Here's how the part is built. I have some questions about the finished solid (model axes, mm). A direction names the side the tool comes from. Give positions to 0.01 mm unless a question says otherwise; leave off trailing zeros. Loops run counter-clockwise (first coordinate to the right, second up) from the corner with the lowest first, then second, coordinate; pieces in that order, holes last. Notation, with made-up numbers: (61, 27.5) - (72, 27.5) arc R13 ccw to (72, 48.5) - close; hole circle Ø1 at (-30.5, -10). An arc over 180 degrees is marked (long way). Put each result on its own line as item: value. Start each with the question number.
from build123d import *

# Parameters (mm, degrees)
ESQUISSE1_W             = 5
ESQUISSE1_H             = 40
BOSS_EXTRU_1_DEPTH      = 10
ESQUISSE2_R             = 2.6
ENL_V_MAT_EXTRU_1_DEPTH = 10
ESQUISSE3_W             = 5
ESQUISSE3_H             = 40
BOSS_EXTRU_2_DEPTH      = 6
CONG_1_R                = 7
ESQUISSE6_W             = 3
ESQUISSE6_H             = 33
BOSS_EXTRU_4_DEPTH      = 120
ESQUISSE8_R             = 2.6
BOSS_EXTRU_5_DEPTH      = 5
ESQUISSE9_W             = 130
ESQUISSE9_H             = 3
ENL_V_MAT_EXTRU_2_DEPTH = 20


with BuildPart() as part:
    # Esquisse1 → Boss.-Extru.1 (new body)
    with BuildSketch(Plane.XY):
        with Locations((2.5, -20)):
            Rectangle(ESQUISSE1_W, ESQUISSE1_H)
    extrude(amount=BOSS_EXTRU_1_DEPTH)

    # Esquisse2 → Enlèv. mat.-Extru.1 (cut)
    with BuildSketch(Plane(origin=(5, 0, 0), x_dir=(0, 0, -1), z_dir=(1, 0, 0))):
        with Locations((-5, -35)):
            Circle(ESQUISSE2_R)
    extrude(amount=-ENL_V_MAT_EXTRU_1_DEPTH, mode=Mode.SUBTRACT)

    # Esquisse3 → Boss.-Extru.2 (add)
    with BuildSketch(Plane.XY.offset(10)):
        with Locations((2.5, -20)):
            Rectangle(ESQUISSE3_W, ESQUISSE3_H)
    extrude(amount=BOSS_EXTRU_2_DEPTH)

    # Congé1
    cong_1_edges = [part.edges().sort_by_distance(p)[0] for p in [
        (2.5, -40, 16),
    ]]
    fillet(cong_1_edges, radius=CONG_1_R)

    # Esquisse6 → Boss.-Extru.4 (add)
    with BuildSketch(Plane.ZY):
        with Locations((14.5, -16.5)):
            Rectangle(ESQUISSE6_W, ESQUISSE6_H)
    extrude(amount=BOSS_EXTRU_4_DEPTH)

    # Esquisse8 → Boss.-Extru.5 (add)
    with BuildSketch(Plane.ZY.offset(120)):
        with BuildLine():
            Line((16, 0), (0, 0))
            Line((0, 0), (0, -40))
            Line((0, -40), (9, -40))
            ThreePointArc((9, -40), (13.949747468, -37.949747468), (16, -33))
            Line((16, -33), (16, 0))
        make_face()
        with Locations((5, -35)):
            Circle(ESQUISSE8_R, mode=Mode.SUBTRACT)
    extrude(amount=BOSS_EXTRU_5_DEPTH)

    # Esquisse9 → Enlèv. mat.-Extru.2 (cut)
    with BuildSketch(Plane.XY):
        with Locations((-60, -1.5)):
            Rectangle(ESQUISSE9_W, ESQUISSE9_H)
    extrude(amount=ENL_V_MAT_EXTRU_2_DEPTH, mode=Mode.SUBTRACT)


solid = part.part
1) Suppose I cut it at B-B on y = -35. Please give me the cut outline in (x, z).
2) Suppose I cut it at A-A on z = 5. Please give me the cut outline in (x, y).
3) Suppose I cut it at C-C on y = -26.5. Please give me the cut outline in (x, z).
4) Which directions (+Z, -Z, +X, -X, +Y, -Y) give clear straight access to the entire face, cutting with the end or side of a thin tool? Please do faces 1 (the flat face through (-59, -18, 13)), 2 (the flat face through (-59, -33, 14)), 3 (the cylindrical face through (-122.5, -38, 13.9)).
5) I'm going to push flat-ended pins straight in: P1, Ø1.5, axis at x = -99.5, y = -31, coming from the -Z side; P2, Ø3, axis at x = -91, z = 13, coming from the -Y side; P3, Ø4, axis at y = -35, z = 5, coming from the +X side. Where does each tip first touch, or does it pass through?
6) Thinking about a two-plate mould opening in Y: for faces 4 (the flat face through (-122, -40, 4)), 5 (the flat face through (-120, -21, 6)), 6 (the cylindrical face through (2.54, -34.22, 2.52)), which applies, pulls with the +Y half, pulls with the -Y half, needs draft (parallel to the pull), parting line crosses it, or undercut?
7) I need wall thicknesses on line 1 (X direction, y = -20.5, z = 8.75); line 2 (Y direction, x = -122.9, z = 5); line 3 (Z direction, x = -83, y = -10). Which ranges of each line are inside material? Lowest first, please.
8) Suppose I cut it at D-D on x = -62. Please give me the cut outline in (y, z), plus the area to 3 significant figures.
Ans:
1. outline: (-125, 0) - (-120, 0) - (-120, 2.4) - (-125, 2.4) - close; (-125, 7.6) - (-120, 7.6) - (-120, 15.71) - (-125, 15.71) - close; (0, 0) - (5, 0) - (5, 2.4) - (0, 2.4) - close; (0, 7.6) - (5, 7.6) - (5, 15.71) - (0, 15.71) - close
2. outline: (-125, -40) - (-120, -40) - (-120, -37.6) - (-125, -37.6) - close; (-125, -32.4) - (-120, -32.4) - (-120, -3) - (-125, -3) - close; (0, -40) - (5, -40) - (5, -37.6) - (0, -37.6) - close; (0, -32.4) - (5, -32.4) - (5, -3) - (0, -3) - close
3. outline: (-125, 0) - (-120, 0) - (-120, 13) - (0, 13) - (0, 0) - (5, 0) - (5, 16) - (-125, 16) - close
4. face 1: -Z, +Y, -Y
4. face 2: +Z, -Z, -Y
4. face 3: +Z, +X, -X, -Y
5. P1: stops at z = 13
5. P2: stops at y = -33
5. P3: passes through
6. face 4: pulls with the -Y half
6. face 5: needs draft
6. face 6: undercut
7. line 1: x = -125 to -120, 0 to 5
7. line 2: y = -40 to -37.6, -32.4 to -3
7. line 3: z = 13 to 16
8. outline: (-33, 13) - (-3, 13) - (-3, 16) - (-33, 16) - close
8. area: 90.0 mm²
